Build history of the part. All positions in model axes, mm. A direction names the side the tool comes from. Give positions to 0.01 mm unless a question says otherwise; leave off trailing zeros. Order: outer loops, then holes, each group sorted by start corner. A loop starts at its lowest first (then second) coordinate and runs counter-clockwise, first axis right, second up. Notation, with made-up numbers: (76, -1) - (94, -1) arc R32 cw to (94, 26) - close; hole circle Ø5 at (-32, 25). An arc over 180 degrees is marked (long way). One line per item, written item: value.
```python
from build123d import *
from build123d.topology import SkipClean

# Parameters (mm, degrees)
SKETCH1_R           = 3.175
SKETCH1_R_2         = 1.5875
BOSS_EXTRUDE1_DEPTH = 4.7625
SKETCH2_R           = 0.79375
BOSS_EXTRUDE2_DEPTH = 1.5875


with BuildPart() as part:
    # Sketch1 → Boss-Extrude1 (new body)
    with BuildSketch(Plane.XY):
        with Locations(Location((14.60119787, -1.564197578, 0), (0, 0, 180))):
            Circle(SKETCH1_R)
        with Locations(Location((14.60119787, -1.564197578, 0), (0, 0, 180))):
            Circle(SKETCH1_R_2, mode=Mode.SUBTRACT)
    extrude(amount=BOSS_EXTRUDE1_DEPTH)

    # Sketch2 → Boss-Extrude2 (add)
    with SkipClean():  # the faces are left unmerged after this step: merging them gives an invalid solid
        with BuildSketch(Plane.XY.offset(4.7625)):
            with BuildLine():
                Line((11.465194702, -1.068103704), (13.033196686, 8.843849359))
                ThreePointArc((13.033196686, 8.843849359), (14.60119833, 10.183302422), (16.169199873, 8.843849241))
                Line((16.169199873, 8.843849241), (17.737201077, -1.068103951))
                ThreePointArc((17.737201077, -1.068103951), (14.601197744, -4.739197578), (11.465194702, -1.068103704))
            make_face()
            with Locations((14.60119827, 8.595802422)):
                Circle(SKETCH2_R, mode=Mode.SUBTRACT)
        extrude(amount=BOSS_EXTRUDE2_DEPTH)


solid = part.part
```
(1) Drill centre lines: line 1 (Y direction, x = 14.5, z = 1); line 2 (Z direction, x = 16.25, y = 7); line 3 (X direction, y = -3, z = 1). Where is each one in solid material? Low to high.
Completed:
line 1: -4.74 to -3.15, 0.02 to 1.61
line 2: 4.76 to 6.35
line 3: 11.77 to 13.92, 15.28 to 17.43
(2) 3-axis set-ups, long thin cutter, end or side, ignore diameter. For faces 4 (the face through (12.24, 3.82, 5.55)), 5 (the face through (16.187, -1.634, 2.348)): which of +Z, -Z, +X, -X, +Y, -Y reach the whole face in a straight line?
Completed:
face 4: +Z, -Z, -X, +Y
face 5: -Z
(3) Slice it at D-D, the plane x = 12.5. Give the cut face in (y, z).
Completed:
outline: (-3.94, 0) - (0.82, 0) - (0.82, 4.76) - (5.47, 4.76) - (5.47, 6.35) - (-3.94, 6.35) - close
(4) Slice it at A-A, the plane x = 14. Give the cut face in (y, z), and give its area (3 significant figures).
Completed:
outline: (-4.68, 0) - (-3.03, 0) - (-3.03, 4.76) - (-0.09, 4.76) - (-0.09, 0) - (1.55, 0) - (1.55, 4.76) - (8.08, 4.76) - (8.08, 6.35) - (-4.68, 6.35) - close; (9.11, 4.76) - (10.07, 4.76) - (10.07, 6.35) - (9.11, 6.35) - close
area: 37.5 mm²
(5) Slice it at B-B, the plane y = 8. Give the cut face in (x, z).
Completed:
outline: (12.9, 4.76) - (14.08, 4.76) - (14.08, 6.35) - (12.9, 6.35) - close; (15.13, 4.76) - (16.3, 4.76) - (16.3, 6.35) - (15.13, 6.35) - close
(6) Pull direction Y, two halves, no side cores. Call faces 1 (the face through (15, -2, 4.762)), 2 (the face through (15, 1, 6.35)), 3 (the face through (16.94, 3.96, 5.55)): +Y half, -Y half, draft (parallel to the pull), parting line (faces both ways), or undercut.
Completed:
face 1: undercut
face 2: draft
face 3: +Y half
(7) Pin check, flat tips, straight feed: P1, Ø3, axis at x = 15, z = 3, coming from the +Y side; P2, Ø2, axis at x = 16, z = 5.5, coming from the -Y side; P3, Ø2, axis at x = 14.6, y = 8.6, coming from the -Z side. Stop position of each tip, or through.
Completed:
P1: y = 1.61
P2: y = -4.71
P3: z = 4.76
